The listing builds one solid part. Answer for the finished solid, in the listing's coordinates (mm). Face numbers are marked on the shaded views. Round coordinates to 2 decimals unless told otherwise and drop trailing zeros. Write each loop counter-clockwise with the first axis right and the second up, starting at its lowest first coordinate (ties: lowest second). Pieces come first, ordered by that corner, then holes. Notation, with made-up numbers: (86.5, -9.5) -> (107.5, -9.5) arc R21 cw to (107.5, 12.5) -> close; hole circle Ø6 at (-32.75, 27.25). An arc over 180 degrees is marked (long way). Write each question's results on one line, items separated by ' | '. Start each with the question number.
```python
from build123d import *

# Parameters (mm, degrees)
F0_R     = 16
F1_DEPTH = 165
F4_R     = 11
F7_R     = 23
F8_DEPTH = 5


with BuildPart() as f1:
    # F0 (on Top) → F1 (new body)
    with BuildSketch(Plane.XY):
        Circle(F0_R)
    extrude(amount=F1_DEPTH)

    # F6: sweep along a path in F5
    with BuildLine(Plane.XZ) as f6_path:
        Line((0, 116.2202451894), (83.9946197184, 116.2202451894))
        Line((83.9946197184, 116.2202451894), (120, 60))
    # F4 (on Right) → F6 (sweep)
    with BuildSketch(Plane.YZ):
        with Locations((0, 116.2202451894)):
            Circle(F4_R)
    sweep(path=f6_path.line, transition=Transition.RIGHT)

    # F7 (on Top) → F8 (join)
    with BuildSketch(Plane.XY):
        Circle(F7_R)
    extrude(amount=F8_DEPTH)


solid = f1.part
```
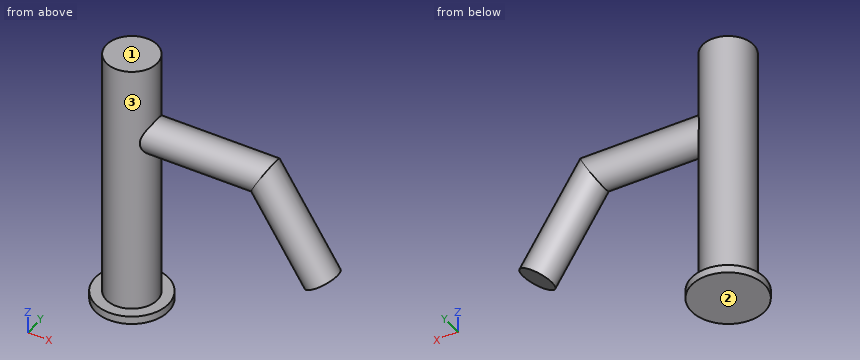
Q1. Determine the mould class of the marked faces 1, 2 and 3 for opening direction Z: pulls with the +Z half, pulls with the -Z half, needs draft (parallel to the pull), parting line crosses it, or undercut.
Q2. The part is cut by section C-C, the plane z = 25.5. Write down the section's boundary in (x, y).
Q3. The part is cut by section B-B, the plane x = 0. Write down the section's boundary in (y, z).
Q4. Each of these flat-tipped pins is pushed along its axis until it touches: pin 1 (1 mm diameter, centred on y = 15, z = 68.5, fed in from +X); pin 2 (1 mm diameter, centred on x = 97, z = 96, fed in from +Y); pin 3 (12 mm diameter, centred on x = 45, y = 0, fed in from -Z). Where does it stop, or does it pass through?
Q5. The part is cut by section A-A, the plane y = 0. Write down the section's boundary in (x, z).
Q6. The part is cut by section D-D, the plane x = 21. Write down the section's boundary in (y, z), then the cut area to 3 significant figures.
Q7. Find the intervals of material crossed by line 1 (Z direction, x = 18.5, y = -1); line 2 (Y direction, x = 78, z = 116.5); line 3 (Z direction, x = 1, y = -17.5), in increasing order.
Answers follow:
1) face 1: pulls with the +Z half | face 2: pulls with the -Z half | face 3: undercut
2) outline: circle Ø32 at (0, 0)
3) outline: (-23, 0) -> (23, 0) -> (23, 5) -> (16, 5) -> (16, 165) -> (-16, 165) -> (-16, 5) -> (-23, 5) -> close
4) pin 1: x = 6.76 | pin 2: y = 11 | pin 3: z = 105.22
5) outline: (-23, 0) -> (23, 0) -> (23, 5) -> (16, 5) -> (16, 105.22) -> (77.98, 105.22) -> (110.74, 54.07) -> (129.26, 65.93) -> (90.01, 127.22) -> (16, 127.22) -> (16, 165) -> (-16, 165) -> (-16, 5) -> (-23, 5) -> close
6) outline: circle Ø22 at (0, 116.22); (-9.38, 0) -> (9.38, 0) -> (9.38, 5) -> (-9.38, 5) -> close | area: 474 mm^2
7) line 1: 0 to 5, 105.27 to 127.17 | line 2: -11 to 11 | line 3: 0 to 5
